Read the model definition and answer for the solid it produces. Units are mm, in the model's axes. A direction names the side the tool comes from. Coordinates: 2 decimals unless noted, no trailing zeros. Write each loop counter-clockwise with the first axis right and the second up, starting at its lowest first coordinate (ties: lowest second). Pieces come first, ordered by that corner, then holes.
(1) Section A-A on y = 30.25 is taken. Write down the section's boundary in (x, z).
(2) Find the intervals of material crossed by probe 1 along Z at (x, y) = (118.25, 31.5); probe 2 along Y at (x, z) = (118.55, 79.5); probe 3 along Y at (x, z) = (118.1, 96), in increasing order.
(3) Which of the six approach directions +Z, -Z, +X, -X, +Y, -Y give full straight-line access (tool end or side, diameter ignored) to faces 1 (the flat face through (118.5, 30.3, 111)), 2 (the cylindrical face through (118.493, 19.346, 111.184))?
(4) Given pin 1 (0.5 mm diameter, centred on x = 118.5, z = 93.5, fed in from -Y), flat-ended and moving along its own axis, determine where the tip first touches the part or whether it passes through.
(5) The mould has two halves that part along Z. Classify faces 3 (the cylindrical face through (118.493, 18.911, 75.746)), 4 (the flat face through (118.5, 30.3, 112)), 5 (the cylindrical face through (118.507, 40.248, 75.713)), 6 (the cylindrical face through (118.51, 41.1, 74.86)): +Z half, -Z half, draft (parallel to the pull), parting line (faces both ways), or undercut.
(6) Section B-B on z = 109.5 is taken. Write down the section's boundary in (x, y).
(7) Section C-C on x = 118.45 is taken. Write down the section's boundary in (y, z), then the cut area to 3 significant figures.
from build123d import *

# Parameters (mm, degrees)
BOX055_W          = 5
BOX055_H          = 24
BOX055_DEPTH      = 40
BOX055_ROLL_ANGLE = -2.2
BOX054_W          = 1
BOX054_H          = 23
BOX054_DEPTH      = 36
FILLET061_R       = 2.5
BOX011_W          = 5
BOX011_H          = 24
BOX011_DEPTH      = 40
BOX011_ROLL_ANGLE = -2.2
BOX010_W          = 1
BOX010_H          = 25
BOX010_DEPTH      = 38
FILLET047_R       = 3


with BuildPart() as cube481:
    # Box055 → Box055 (new body)
    with BuildSketch(Plane.XY):
        with Locations((2.5, 12)):
            Rectangle(BOX055_W, BOX055_H)
    extrude(amount=BOX055_DEPTH)


with BuildPart() as cube481_1:
    # Box055 roll: moved
    add(cube481.part.rotate(Axis((0, 0, 0), (1, 0, 0)), BOX055_ROLL_ANGLE))


with BuildPart() as cube481_2:
    # Box055 placement: moved
    add(cube481_1.part.moved(Location((175, -23, -1))))


with BuildPart() as fillet061:
    # Box054 → Box054 (new body)
    with BuildSketch(Plane(origin=(175, 1, 1), x_dir=(1, 0, 0), z_dir=(0, 0, 1))):
        with Locations((0.5, 11.5)):
            Rectangle(BOX054_W, BOX054_H)
    extrude(amount=BOX054_DEPTH)

    # Cut040: cut Cube481
    add(cube481_2.part, mode=Mode.SUBTRACT)


with BuildPart() as fillet061_1:
    # Cut040 placement: moved
    add(fillet061.part.moved(Location((-57, 17, 74))))

    # Fillet061
    fillet061_edges = [fillet061_1.edges().sort_by_distance(p)[0] for p in [
        (118.5, 41, 111),
        (118.5, 19.477516, 111),
        (118.5, 41, 75),
        (118.5, 18.094535, 75),
    ]]
    fillet(fillet061_edges, radius=FILLET061_R)


with BuildPart() as cube379:
    # Box011 → Box011 (new body)
    with BuildSketch(Plane.XY):
        with Locations((2.5, 12)):
            Rectangle(BOX011_W, BOX011_H)
    extrude(amount=BOX011_DEPTH)


with BuildPart() as cube379_1:
    # Box011 roll: moved
    add(cube379.part.rotate(Axis((0, 0, 0), (1, 0, 0)), BOX011_ROLL_ANGLE))


with BuildPart() as cube379_2:
    # Box011 placement: moved
    add(cube379_1.part.moved(Location((175, -24, -1))))


with BuildPart() as cut041:
    # Box010 → Box010 (new body)
    with BuildSketch(Plane(origin=(175, 0, 0), x_dir=(1, 0, 0), z_dir=(0, 0, 1))):
        with Locations((0.5, 12.5)):
            Rectangle(BOX010_W, BOX010_H)
    extrude(amount=BOX010_DEPTH)

    # Cut004: cut Cube379
    add(cube379_2.part, mode=Mode.SUBTRACT)


with BuildPart() as cut041_1:
    # Cut004 placement: moved
    add(cut041.part.moved(Location((-57, 17, 74))))

    # Fillet047
    fillet047_edges = [cut041_1.edges().sort_by_distance(p)[0] for p in [
        (118.5, 42, 112),
        (118.5, 18.515932, 112),
        (118.5, 42, 74),
        (118.5, 17.056119, 74),
    ]]
    fillet(fillet047_edges, radius=FILLET047_R)

    # Cut041: cut Fillet061
    add(fillet061_1.part, mode=Mode.SUBTRACT)


solid = cut041_1.part
Response:
1. outline: (118, 74) - (119, 74) - (119, 75) - (118, 75) - close; (118, 111) - (119, 111) - (119, 112) - (118, 112) - close
2. probe 1: z = 74 to 75, 111 to 112
2. probe 2: y = 17.27 to 18.27, 41 to 42
2. probe 3: y = 17.9 to 18.9, 41 to 42
3. face 1: +X, -X
3. face 2: +Z, +X, -X, -Y
4. pin 1: stops at y = 17.8
5. face 3: undercut
5. face 4: +Z half
5. face 5: undercut
5. face 6: -Z half
6. outline: (118, 18.44) - (119, 18.44) - (119, 19.59) - (118, 19.59) - close; (118, 40.79) - (119, 40.79) - (119, 41.96) - (118, 41.96) - close
7. outline: (17.18, 77.12) arc R3 ccw to (20.17, 74) - (39, 74) arc R3 ccw to (42, 77) - (42, 109) arc R3 ccw to (39, 112) - (21.4, 112) arc R3 ccw to (18.41, 109.12) - close; hole (18.19, 77.6) arc R2.5 ccw to (20.69, 75) - (38.5, 75) arc R2.5 ccw to (41, 77.5) - (41, 108.5) arc R2.5 ccw to (38.5, 111) - (21.88, 111) arc R2.5 ccw to (19.39, 108.6) - close
7. area: 118 mm2
